Verification items for the finished model (mm, model axes). A direction names the side the tool comes from. Coordinates: 2 decimals unless noted, no trailing zeros. Write each loop counter-clockwise with the first axis right and the second up, starting at its lowest first coordinate (ties: lowest second). Pieces come first, ordered by that corner, then holes. Notation, with made-up numbers: (-37.75, -31) -> (-22.75, -31) arc R21 cw to (-22.75, 4) -> close; hole circle Ø10 at (-27.75, -12.5). An arc over 180 degrees is marked (long way). Answer in a Markdown table with one row per item.
```python
from build123d import *

# Parameters (mm, degrees)
SKETCH2_W           = 69.549132125
SKETCH2_H           = 18.652417492
SKETCH2_R           = 3.792348853
BOSS_EXTRUDE1_DEPTH = 6.35


with BuildPart() as part:
    # Sketch2 → Boss-Extrude1 (new body)
    with BuildSketch(Plane.ZY):
        with Locations((13.384474921, 36.326123608)):
            Rectangle(SKETCH2_W, SKETCH2_H)
        with Locations((-12.28496421, 36.326123608)):
            Circle(SKETCH2_R, mode=Mode.SUBTRACT)
        Polygon((-2.169792441, 30.018483291), (-2.169792441, 35.496966931), (37.864979034, 35.496966931), (37.864979034, 37.355942436), (34.900155127, 37.355942436), (34.900155127, 42.834426076), (43.343462674, 42.834426076), (43.343462674, 30.018483291), (37.864979034, 30.018483291), align=None, mode=Mode.SUBTRACT)
    extrude(amount=BOSS_EXTRUDE1_DEPTH)


solid = part.part
```
1. Material ranges on probe 1 along Y at (x, z) = (-0.75, 37.5); probe 2 along Z at (x, y) = (-1.75, 36); probe 3 along Y at (x, z) = (-0.5, 5), recorded low to high. Write a range as from..to.
Findings below:
| item | result |
|---|---|
| probe 1 | y = 27..30.02, 35.5..37.36, 42.83..45.65 |
| probe 2 | z = -21.39..-16.06, -8.51..37.86, 43.34..48.16 |
| probe 3 | y = 27..30.02, 35.5..45.65 |
2. Sectioned sample at C-C, the plane x = -5.5. Record the cut outline in (y, z).
Findings below:
| item | result |
|---|---|
| outline | (27, -21.39) -> (45.65, -21.39) -> (45.65, 48.16) -> (27, 48.16) -> close; hole (30.02, -2.17) -> (35.5, -2.17) -> (35.5, 37.86) -> (37.36, 37.86) -> (37.36, 34.9) -> (42.83, 34.9) -> (42.83, 43.34) -> (30.02, 43.34) -> close; hole circle Ø7.58 at (36.33, -12.28) |
3. Sectioned sample at A-A, the plane z = 41. Record the cut outline in (x, y), and give its area (3 significant figures).
Findings below:
| item | result |
|---|---|
| outline | (-6.35, 27) -> (0, 27) -> (0, 30.02) -> (-6.35, 30.02) -> close; (-6.35, 42.83) -> (0, 42.83) -> (0, 45.65) -> (-6.35, 45.65) -> close |
| area | 37.1 mm² |
4. Access from +Z, -Z, +X, -X, +Y, -Y to the whole of each face (thin tool, end or side, straight path). Record for faces 4 (the face through (-3, 36, 48.159)), 5 (the face through (-3, 37.356, 36)).
Findings below:
| item | result |
|---|---|
| face 4 | +Z, +X, -X, +Y, -Y |
| face 5 | +X, -X |
5. Sectioned sample at B-B, the plane y = 39. Record the cut outline in (x, z).
Findings below:
| item | result |
|---|---|
| outline | (-6.35, -21.39) -> (0, -21.39) -> (0, -14.97) -> (-6.35, -14.97) -> close; (-6.35, -9.6) -> (0, -9.6) -> (0, 34.9) -> (-6.35, 34.9) -> close; (-6.35, 43.34) -> (0, 43.34) -> (0, 48.16) -> (-6.35, 48.16) -> close |
6. Sectioned sample at D-D, the plane z = 32. Record the cut outline in (x, y), and give its area (3 significant figures).
Findings below:
| item | result |
|---|---|
| outline | (-6.35, 27) -> (0, 27) -> (0, 30.02) -> (-6.35, 30.02) -> close; (-6.35, 35.5) -> (0, 35.5) -> (0, 45.65) -> (-6.35, 45.65) -> close |
| area | 83.7 mm² |
7. Release check for a two-part mould opening along Z. For faces 1 (the face through (-3, 45.652, 13)), 2 (the face through (-3, 36, -21.39)), 3 (the face through (-3, 42.834, 39)) record: released by +Z, released by -Z, zero draft, split by the parting line, or undercut.
Findings below:
| item | result |
|---|---|
| face 1 | zero draft |
| face 2 | released by -Z |
| face 3 | undercut |
